Here's how the part is built. I have some questions about the finished solid (model axes, mm). A direction names the side the tool comes from. Coordinates: 2 decimals unless noted, no trailing zeros. Order: outer loops, then holes, each group sorted by start corner. A loop starts at its lowest first (then second) coordinate and runs counter-clockwise, first axis right, second up. Notation, with made-up numbers: (-25, 25.5) - (-9, 25.5) arc R20 ccw to (-9, 38.5) - close; hole circle Ø3 at (-3.5, -8). An arc over 180 degrees is marked (long way). Use CSV: the item, a comma, the result in double quotes. Start each with the question number.
from build123d import *

# Parameters (mm, degrees)
SKETCH_1_R          = 18.5
EXTRUDE_1_DEPTH     = 24
SKETCH_1_3_R        = 1.5
CUT_EXTRUDE_1_DEPTH = 20
SKETCH_3_R          = 16.4
EXTRUDE_3_DEPTH     = 22
SKETCH_4_R          = 6
EXTRUDE_4_DEPTH     = 6
SKETCH_5_R          = 3
EXTRUDE_5_DEPTH     = 3
EXTRUDE_6_DEPTH     = 12
SKETCH_7_R          = 15
EXTRUDE_7_DEPTH     = 1
SKETCH_8_R          = 16.5
EXTRUDE_8_DEPTH     = 2
SKETCH_9_R          = 6.5
EXTRUDE_9_DEPTH     = 6


with BuildPart() as part:
    # 草图1 → 凸台-拉伸1 (new body)
    with BuildSketch(Plane.XY):
        Circle(SKETCH_1_R)
    extrude(amount=EXTRUDE_1_DEPTH)

    # 草图1<3> → 切除-拉伸1 (cut)
    with BuildSketch(Plane.XY):
        with Locations((-15.5, 0)):
            Circle(SKETCH_1_3_R)
        with Locations((-7.75, 13.423393759)):
            Circle(SKETCH_1_3_R)
        with Locations((-7.75, -13.423393759)):
            Circle(SKETCH_1_3_R)
        with Locations((7.75, 13.423393759)):
            Circle(SKETCH_1_3_R)
        with Locations((15.5, 0)):
            Circle(SKETCH_1_3_R)
        with Locations((7.75, -13.423393759)):
            Circle(SKETCH_1_3_R)
    extrude(amount=CUT_EXTRUDE_1_DEPTH, mode=Mode.SUBTRACT)

    # 草图3 → 凸台-拉伸3 (add)
    with BuildSketch(Plane.XY.offset(24)):
        Circle(SKETCH_3_R)
    extrude(amount=EXTRUDE_3_DEPTH)

    # 草图4 → 凸台-拉伸4 (add)
    with BuildSketch(Plane(origin=(0, 0, 0), x_dir=(-1, 0, 0), z_dir=(0, 0, -1))):
        with Locations(Location((0, 7, 0), (0, 0, 180))):
            Circle(SKETCH_4_R)
    extrude(amount=EXTRUDE_4_DEPTH)

    # 草图5 → 凸台-拉伸5 (add)
    with BuildSketch(Plane(origin=(0, 0, -6), x_dir=(-1, 0, 0), z_dir=(0, 0, -1))):
        with Locations((0, 7)):
            Circle(SKETCH_5_R)
    extrude(amount=EXTRUDE_5_DEPTH)

    # 草图6 → 凸台-拉伸6 (add)
    with BuildSketch(Plane(origin=(0, 0, -9), x_dir=(-1, 0, 0), z_dir=(0, 0, -1))):
        with BuildLine():
            Line((-1.8, 9.4), (1.8, 9.4))
            ThreePointArc((1.8, 9.4), (0, 4), (-1.8, 9.4))
        make_face()
    extrude(amount=EXTRUDE_6_DEPTH)

    # 草图7 → 凸台-拉伸7 (add)
    with BuildSketch(Plane.XY.offset(46)):
        Circle(SKETCH_7_R)
    extrude(amount=EXTRUDE_7_DEPTH)

    # 草图8 → 凸台-拉伸8 (add)
    with BuildSketch(Plane.XY.offset(47)):
        Circle(SKETCH_8_R)
    extrude(amount=EXTRUDE_8_DEPTH)

    # 草图9 → 凸台-拉伸9 (add)
    with BuildSketch(Plane.XY.offset(49)):
        Circle(SKETCH_9_R)
        with BuildLine():
            Line((-2, 10), (2, 10))
            ThreePointArc((2, 10), (2.353553391, 9.853553391), (2.5, 9.5))
            Line((2.5, 9.5), (2.5, 8.5))
            ThreePointArc((2.5, 8.5), (2.353553391, 8.146446609), (2, 8))
            Line((2, 8), (-2, 8))
            ThreePointArc((-2, 8), (-2.353553391, 8.146446609), (-2.5, 8.5))
            Line((-2.5, 8.5), (-2.5, 9.5))
            ThreePointArc((-2.5, 9.5), (-2.353553391, 9.853553391), (-2, 10))
        make_face()
        with BuildLine():
            Line((8.5, 2.5), (9.5, 2.5))
            ThreePointArc((9.5, 2.5), (9.853553391, 2.353553391), (10, 2))
            Line((10, 2), (10, -2))
            ThreePointArc((10, -2), (9.853553391, -2.353553391), (9.5, -2.5))
            Line((9.5, -2.5), (8.5, -2.5))
            ThreePointArc((8.5, -2.5), (8.146446609, -2.353553391), (8, -2))
            Line((8, -2), (8, 2))
            ThreePointArc((8, 2), (8.146446609, 2.353553391), (8.5, 2.5))
        make_face()
    extrude(amount=EXTRUDE_9_DEPTH)


solid = part.part
Item 1: For faces 1 (the flat face through (8, 0, 52)), 2 (the flat face through (15, -5, 46)), 3 (the cylindrical face through (-8.856, -12.41, 9.86)), which set-ups out of +Z, -Z, +X, -X, +Y, -Y let a thin tool reach every point of the face, with its end or its side?
Item 2: Suppose I cut it at D-D on z = 10. Write out the boundary of the cut face in (x, y).
Item 3: Suppose I cut it at C-C on z = -2. Write out the boundary of the cut face in (x, y).
Item 4: For pin 1 Ø2.5 at (x, y) = (-15.5, 0) entering from -Z; pin 2 Ø8 at (x, y) = (-3.5, 10) entering from +Z; pin 3 Ø1.5 at (x, y) = (8.5, 13) entering from -Z; pin 4 Ø0.8 at (y, z) = (9, 53) entering from +X, each with a flat end and sliding along its axis, tell me the tip position at first contact or that it passes through.
Item 5: Please list where these lines run through material, in increasing order: line 1 along Y through (x, z) = (7, 15); line 2 along X through (y, z) = (12.5, 16); line 3 along Y through (x, z) = (-7.75, 8.75). Write a range as from..to.
Item 6: We'd pull the mould along Y, two halves only. Please class faces 4 (the cylindrical face through (6.644, -12.41, 9.86)), 5 (the flat face through (0, 0, 55)), 6 (the cylindrical face through (-14.985, 0.66, 46.493)), 7 (the flat face through (-16, 0, 20)): released by +Y, released by -Y, zero draft, split by the parting line, or undercut.
Here are the results:
1,face 1,"+Z, +Y, -Y"
1,face 2,"none"
1,face 3,"-Z"
2,outline,"circle Ø37 at (0, 0); hole circle Ø3 at (-15.5, 0); hole circle Ø3 at (-7.75, -13.42); hole circle Ø3 at (-7.75, 13.42); hole circle Ø3 at (7.75, -13.42); hole circle Ø3 at (7.75, 13.42); hole circle Ø3 at (15.5, 0)"
3,outline,"circle Ø12 at (0, 7)"
4,pin 1,"z = 20"
4,pin 2,"z = 55"
4,pin 3,"z = 0"
4,pin 4,"x = 2.5"
5,line 1,"-17.12..-14.72, -12.12..12.12, 14.72..17.12"
5,line 2,"-13.64..-8.93, -6.57..6.57, 8.93..13.64"
5,line 3,"-16.8..-14.92, -11.92..11.92, 14.92..16.8"
6,face 4,"undercut"
6,face 5,"zero draft"
6,face 6,"split by the parting line"
6,face 7,"undercut"
